from build123d import *

# Parameters (mm, degrees)
F1_DEPTH = 3.5
F3_DEPTH = 115


with BuildPart() as f1:
    # F0 (on Top) → F1 (new body)
    with BuildSketch(Plane.XY):
        with BuildLine():
            Line((82.8955, 28.39768), (-2.3045, 28.39768))
            Line((-2.3045, 28.39768), (-2.3045, -46.80232))
            Line((-2.3045, -46.80232), (81.958594, -46.80232))
            ThreePointArc((81.958594, -46.80232), (82.621087, -46.527906), (82.8955, -45.865413))
            Line((82.8955, -45.865413), (82.8955, 28.39768))
        make_face()
    extrude(amount=F1_DEPTH)

    # F2 (on face) → F3 (join)
    with BuildSketch(Plane.XY.offset(3.5)):
        with BuildLine():
            Line((69.2955, -45.865413), (69.2955, -45.20232))
            Line((69.2955, -45.20232), (-0.7045, -45.20232))
            Line((-0.7045, -45.20232), (-0.7045, 26.79768))
            Line((-0.7045, 26.79768), (81.2955, 26.79768))
            Line((81.2955, 26.79768), (81.2955, -33.20232))
            Line((81.2955, -33.20232), (81.958594, -33.20232))
            ThreePointArc((81.958594, -33.20232), (82.621087, -32.927906), (82.8955, -32.265413))
            Line((82.8955, -32.265413), (82.8955, 28.39768))
            Line((82.8955, 28.39768), (-2.3045, 28.39768))
            Line((-2.3045, 28.39768), (-2.3045, -46.80232))
            Line((-2.3045, -46.80232), (68.358594, -46.80232))
            ThreePointArc((68.358594, -46.80232), (69.021087, -46.527906), (69.2955, -45.865413))
        make_face()
    extrude(amount=F3_DEPTH)


solid = f1.part
Geometry: final body of the model. Coordinates: model frame, mm. A direction names the side the tool comes from. Give positions to 0.01 mm unless a question says otherwise; leave off trailing zeros. Loops run counter-clockwise (first coordinate to the right, second up) from the corner with the lowest first, then second, coordinate; pieces in that order, holes last. Notation, with made-up numbers: (-19.5, 44) - (2.5, 44) arc R9 ccw to (2.5, 56) - close; hole circle Ø2 at (-27, 26). An arc over 180 degrees is marked (long way). One line per question, with ' | ' between items. Start each with the question number.
(1) Contact query for flat-ended pins moving along their axis: pin 1 (0.5 mm diameter, centred on x = 81.5, z = 61, fed in from -Y); pin 2 (12 mm diameter, centred on x = 61, y = -31, fed in from +Z). Output: stop coordinate, or through.
(2) Section query D-D on x = 78.5. Return loops of the section in (y, z).
(3) Ray query, line 1 (X direction, y = 22.5, z = 55); line 2 (Y direction, x = 19, z = 84.5); line 3 (Z direction, x = 17, y = -12.5). Return the intervals inside material, ascending. Write a range as from..to.
(4) Section query A-A on z = 80. Return loops of the section in (x, y), then the cut area to 3 significant figures.
(5) Pull-direction query (Y, two-part tool) for faces 1 (the flat face through (35, -45.202, 60)), 2 (the flat face through (-2.304, -9, 58)), 3 (the flat face through (41, 28.398, 58)); classes: released by +Y, released by -Y, zero draft, split by the parting line, or undercut.
(6) Reachability of faces 4 (the flat face through (81.296, -3, 60)), 5 (the flat face through (-0.704, -10, 60)), 6 (the flat face through (-1, -6, 118.5)) from +Z, -Z, +X, -X, +Y, -Y: full face, straight path, thin tool, end or side. Return the list, or none.
(7) Section query B-B on y = -30. Return loops of the section in (x, z), then the cut area to 3 significant figures.
(8) Section query C-C on x = 45. Return loops of the section in (y, z).
The answers:
1) pin 1: y = -33.2 | pin 2: z = 3.5
2) outline: (-46.8, 0) - (28.4, 0) - (28.4, 118.5) - (26.8, 118.5) - (26.8, 3.5) - (-46.8, 3.5) - close
3) line 1: -2.3..-0.7, 81.3..82.9 | line 2: -46.8..-45.2, 26.8..28.4 | line 3: 0..3.5
4) outline: (-2.3, -46.8) - (68.36, -46.8) arc R0.94 ccw to (69.3, -45.87) - (69.3, -45.2) - (-0.7, -45.2) - (-0.7, 26.8) - (81.3, 26.8) - (81.3, -33.2) - (81.96, -33.2) arc R0.94 ccw to (82.9, -32.27) - (82.9, 28.4) - (-2.3, 28.4) - close | area: 462 mm2
5) face 1: undercut | face 2: zero draft | face 3: released by +Y
6) face 4: +Z, -Y | face 5: +Z | face 6: +Z, +X, -X, +Y, -Y
7) outline: (-2.3, 0) - (82.9, 0) - (82.9, 118.5) - (81.3, 118.5) - (81.3, 3.5) - (-0.7, 3.5) - (-0.7, 118.5) - (-2.3, 118.5) - close | area: 666 mm2
8) outline: (-46.8, 0) - (28.4, 0) - (28.4, 118.5) - (26.8, 118.5) - (26.8, 3.5) - (-45.2, 3.5) - (-45.2, 118.5) - (-46.8, 118.5) - close
